```python
from build123d import *

# Parameters (mm, degrees)
BOX004_W          = 1.3
BOX004_H          = 3.3
BOX004_DEPTH      = 10
BOX003_W          = 1.3
BOX003_H          = 3.3
BOX003_DEPTH      = 10
CYLINDER004_R     = 1
CYLINDER004_DEPTH = 10
CYLINDER003_R     = 1
CYLINDER003_DEPTH = 10
CYLINDER001_R     = 2.5
CYLINDER001_DEPTH = 4
CYLINDER_R        = 5.9
CYLINDER_DEPTH    = 4
BOX002_W          = 11.8
BOX002_H          = 32.4
BOX002_DEPTH      = 2.5
BOX001_W          = 11.8
BOX001_H          = 22.5
BOX001_DEPTH      = 22.7


with BuildPart() as cubo004:
    # Box004 → Box004 (new body)
    with BuildSketch(Plane(origin=(5.25, 25, 12), x_dir=(1, 0, 0), z_dir=(0, 0, 1))):
        with Locations((0.65, 1.65)):
            Rectangle(BOX004_W, BOX004_H)
    extrude(amount=BOX004_DEPTH)


with BuildPart() as obj1:
    # Box003 → Box003 (new body)
    with BuildSketch(Plane(origin=(5.25, -6, 12), x_dir=(1, 0, 0), z_dir=(0, 0, 1))):
        with Locations((0.65, 1.65)):
            Rectangle(BOX003_W, BOX003_H)
    extrude(amount=BOX003_DEPTH)

    # Fusion005: union Cubo004
    add(cubo004.part)


with BuildPart() as taladro2:
    # Cylinder004 → Cylinder004 (new body)
    with BuildSketch(Plane(origin=(5.9, 24.85, 11), x_dir=(1, 0, 0), z_dir=(0, 0, 1))):
        Circle(CYLINDER004_R)
    extrude(amount=CYLINDER004_DEPTH)


with BuildPart() as taladros001:
    # Cylinder003 → Cylinder003 (new body)
    with BuildSketch(Plane(origin=(5.9, -2.35, 11), x_dir=(1, 0, 0), z_dir=(0, 0, 1))):
        Circle(CYLINDER003_R)
    extrude(amount=CYLINDER003_DEPTH)

    # Fusion004: union Taladro2
    add(taladro2.part)

    # Fusion006: union obj1
    add(obj1.part)


with BuildPart() as cilindro001:
    # Cylinder001 → Cylinder001 (new body)
    with BuildSketch(Plane(origin=(5.9, 10.3, 22.7), x_dir=(1, 0, 0), z_dir=(0, 0, 1))):
        Circle(CYLINDER001_R)
    extrude(amount=CYLINDER001_DEPTH)


with BuildPart() as fusion001:
    # Cylinder → Cylinder (new body)
    with BuildSketch(Plane(origin=(5.9, 16.6, 22.7), x_dir=(1, 0, 0), z_dir=(0, 0, 1))):
        Circle(CYLINDER_R)
    extrude(amount=CYLINDER_DEPTH)

    # Fusion001: union Cilindro001
    add(cilindro001.part)


with BuildPart() as cubo002:
    # Box002 → Box002 (new body)
    with BuildSketch(Plane(origin=(0, -4.7, 15.9), x_dir=(1, 0, 0), z_dir=(0, 0, 1))):
        with Locations((5.9, 16.2)):
            Rectangle(BOX002_W, BOX002_H)
    extrude(amount=BOX002_DEPTH)


with BuildPart() as cuerpo_con_taladros:
    # Box001 → Box001 (new body)
    with BuildSketch(Plane.XY):
        with Locations((5.9, 11.25)):
            Rectangle(BOX001_W, BOX001_H)
    extrude(amount=BOX001_DEPTH)

    # Fusion: union Cubo002
    add(cubo002.part)

    # Fusion003: union Fusion001
    add(fusion001.part)

    # Cut001: cut Taladros001
    add(taladros001.part, mode=Mode.SUBTRACT)


with BuildPart() as cuerpo_con_taladros_1:
    # Cut001 placement: moved
    add(cuerpo_con_taladros.part.moved(Location((-5.9, 0, 0))))


solid = cuerpo_con_taladros_1.part
```
Model file for the job. Use its own axes, mm. A direction names the side the tool comes from. Round coordinates to 2 decimals unless told otherwise and drop trailing zeros. Order: outer loops, then holes, each group sorted by start corner. A loop starts at its lowest first (then second) coordinate and runs counter-clockwise, first axis right, second up. Notation, with made-up numbers: M 71.5,52 L 83.5,52 A32 ccw 83.5,85 Z; hole C 34,14 d1. An arc over 180 degrees is marked long. Use CSV: the item, a comma, the result in double quotes.
Item 1: Probe probe 1 along X at (y, z) = (24.85, 17); probe 2 along Y at (x, z) = (2, 8.25); probe 3 along Y at (x, z) = (0, 17.6). List the from-to ranges inside material, lowest first.
Worked answers:
probe 1,"-5.9 to -1, 1 to 5.9"
probe 2,"0 to 22.5"
probe 3,"-1.35 to 23.85"
Item 2: Saw through at D-D (x = 3.5). List the corners of the cut face in (y, z).
Worked answers:
outline,"M -4.7,15.9 L 0,15.9 L 0,0 L 22.5,0 L 22.5,15.9 L 27.7,15.9 L 27.7,18.4 L 22.5,18.4 L 22.5,22.7 L 21.35,22.7 L 21.35,26.7 L 11.85,26.7 L 11.85,22.7 L 0,22.7 L 0,18.4 L -4.7,18.4 Z"
Item 3: Saw through at C-C (y = 10.3). List the corners of the cut face in (x, z), plus the area to 3 significant figures.
Worked answers:
outline,"M -5.9,0 L 5.9,0 L 5.9,22.7 L 2.5,22.7 L 2.5,26.7 L -2.5,26.7 L -2.5,22.7 L -5.9,22.7 Z"
area,"288 mm²"
Item 4: Saw through at A-A (y = 24.85). List the corners of the cut face in (x, z), plus the area to 3 significant figures.
Worked answers:
outline,"M -5.9,15.9 L -1,15.9 L -1,18.4 L -5.9,18.4 Z; M 1,15.9 L 5.9,15.9 L 5.9,18.4 L 1,18.4 Z"
area,"24.5 mm²"
Item 5: Saw through at B-B (z = 17.5). List the corners of the cut face in (x, y), plus the area to 3 significant figures.
Worked answers:
outline,"M -5.9,-4.7 L -0.65,-4.7 L -0.65,-3.11 A1 cw long 0.65,-3.11 L 0.65,-4.7 L 5.9,-4.7 L 5.9,27.7 L 0.65,27.7 L 0.65,25.61 A1 cw long -0.65,25.61 L -0.65,27.7 L -5.9,27.7 Z"
area,"372 mm²"
Item 6: Which spindle directions (+Z, -Z, +X, -X, +Y, -Y) get a long thin tool onto all of the face, cutting with end or side? Do faces 1 (the face through (0.65, -4, 17)), 2 (the face through (0, 0, 21)), 3 (the face through (-1.4, 25.1, 18.4)). Say none if no direction does.
Worked answers:
face 1,"+Z, -Z, -Y"
face 2,"+Z, +X, -X, -Y"
face 3,"+Z, +X, -X, +Y"
Item 7: Pin check, flat tips, straight feed: pin 1 (2.5 mm diameter, centred on x = 2.5, y = -2, fed in from -Z); pin 2 (1.5 mm diameter, centred on x = -1, z = 7.5, fed in from -Y); pin 3 (1.2 mm diameter, centred on x = 0, y = 24.85, fed in from +Z); pin 4 (6 mm diameter, centred on x = 4.5, z = 12, fed in from +Y). Stop position of each tip, or through.
Worked answers:
pin 1,"z = 15.9"
pin 2,"y = 0"
pin 3,"through"
pin 4,"y = 22.5"
Item 8: Pull direction Y, two halves, no side cores. Call faces 4 (the face through (0, 22.5, 21)), 5 (the face through (-0.65, -4, 17)), 6 (the face through (0.03, -1.35, 17.13)): released by +Y, released by -Y, zero draft, split by the parting line, or undercut.
Worked answers:
face 4,"released by +Y"
face 5,"zero draft"
face 6,"undercut"
